Verification items for this drawing (mm, ordinates from the low corner). Give positions to 0.01 mm unless a question says otherwise; leave off trailing zeros. Loops run counter-clockwise (first coordinate to the right, second up) from the corner with the lowest first, then second, coordinate; pieces in that order, holes last. Notation, with made-up numbers: (28, -8) -> (67, -8) arc R27 ccw to (67, 21) -> close; hole circle Ø11 at (-2, 10.25). An arc over 180 degrees is marked (long way). Answer as a JSON object with one key per item and string values.
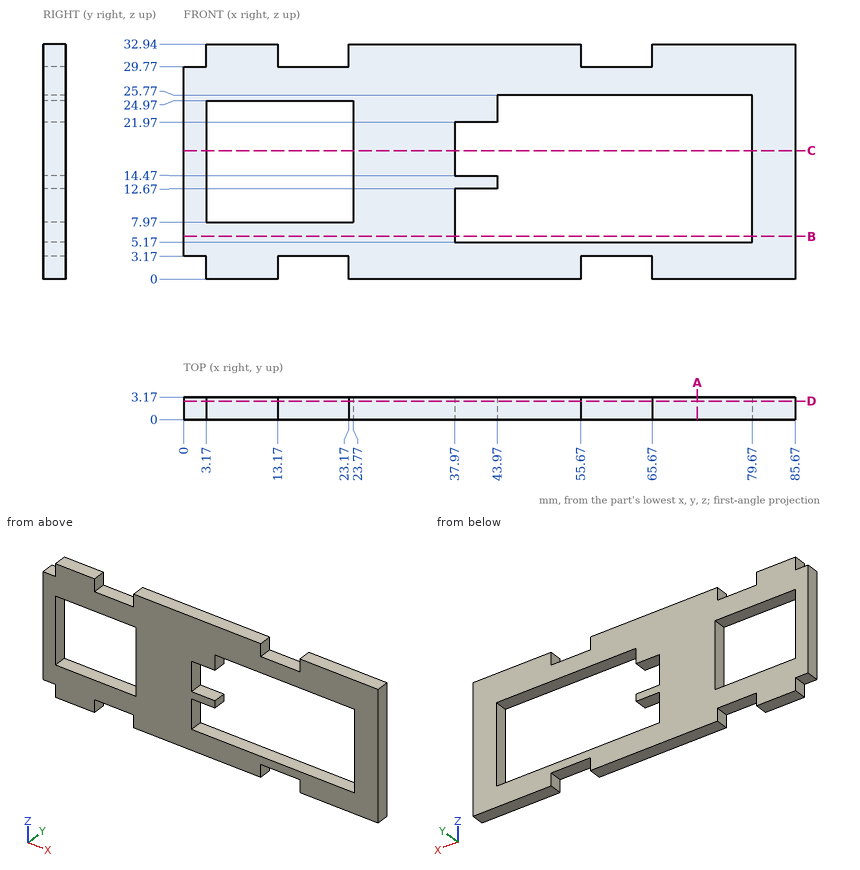
1) Section check D-D on y = 2.6. Count the separate pieces of the cut face and the enclosed holes in it, plus the area to 3 significant figures.
Geometry check:
{"separate pieces": "1", "enclosed holes": "2", "area": "1,500 mm2"}
2) Section check C-C on z = 18. Record the cut outline in (x, y).
Geometry check:
{"outline": "(0, 0) -> (3.17, 0) -> (3.17, 3.17) -> (0, 3.17) -> close; (23.77, 0) -> (37.97, 0) -> (37.97, 3.17) -> (23.77, 3.17) -> close; (79.67, 0) -> (85.67, 0) -> (85.67, 3.17) -> (79.67, 3.17) -> close"}
3) Section check A-A on x = 72. Record the cut outline in (y, z), plus the area to 3 significant figures.
Geometry check:
{"outline": "(0, 0) -> (3.17, 0) -> (3.17, 5.17) -> (0, 5.17) -> close; (0, 25.77) -> (3.17, 25.77) -> (3.17, 32.94) -> (0, 32.94) -> close", "area": "39.1 mm2"}
4) Material ranges on line 1 along X through (y, z) = (2.25, 15.5); line 2 along X through (y, z) = (1, 13.5); line 3 along Z through (x, y) = (61, 2.7), recorded low to high. Write a range as from..to.
Geometry check:
{"line 1": "x = 0..3.17, 23.77..37.97, 79.67..85.67", "line 2": "x = 0..3.17, 23.77..43.97, 79.67..85.67", "line 3": "z = 3.17..5.17, 25.77..29.77"}
5) Depth check by flat-ended pin: P1, Ø1.6, axis at y = 2, z = 31, coming from the -X side; P2, Ø12, axis at x = 69.5, z = 14, coming from the +Y side; P3, Ø1.6, axis at x = 16, y = 2, coming from the -Z side. Enter the tip coordinate at first touch or a pass-through.
Geometry check:
{"P1": "stops at x = 3.17", "P2": "passes through", "P3": "stops at z = 3.17"}
6) Section check B-B on z = 6. Record the cut outline in (x, y), plus the area to 3 significant figures.
Geometry check:
{"outline": "(0, 0) -> (37.97, 0) -> (37.97, 3.17) -> (0, 3.17) -> close; (79.67, 0) -> (85.67, 0) -> (85.67, 3.17) -> (79.67, 3.17) -> close", "area": "139 mm2"}
